from build123d import *

# Parameters (mm, degrees)
SCHIZZO1_R                   = 4
ESTRUSIONE_ESTRUSIONE1_DEPTH = 3
ESTRUSIONE_ESTRUSIONE2_DEPTH = 14
SCHIZZO3_R                   = 1.5
TAGLIO_ESTRUSIONE1_DEPTH     = 32


with BuildPart() as part:
    # Schizzo1 → Estrusione-Estrusione1 (new body)
    with BuildSketch(Plane(origin=(0, 0, 0), x_dir=(1, 0, 0), z_dir=(0, 1, 0))):
        with Locations(Location((0, 0, 0), (0, 0, 270))):
            Circle(SCHIZZO1_R)
    extrude(amount=ESTRUSIONE_ESTRUSIONE1_DEPTH)

    # Schizzo2 → Estrusione-Estrusione2 (add)
    with BuildSketch(Plane(origin=(0, 3, 0), x_dir=(1, 0, 0), z_dir=(0, 1, 0))):
        with BuildLine():
            Line((5.877166346, 8.476701011), (1.77302735, 3.585578617))
            ThreePointArc((1.77302735, 3.585578617), (1.368080573, 3.758770483), (0.94654776, 3.886392587))
            Line((0.94654776, 3.886392587), (0.94654776, 10.271299413))
            Line((0.94654776, 10.271299413), (2, 11.324751653))
            Line((2, 11.324751653), (-2, 11.324751653))
            Line((-2, 11.324751653), (-0.94654776, 10.271299413))
            Line((-0.94654776, 10.271299413), (-0.94654776, 3.886392587))
            ThreePointArc((-0.94654776, 3.886392587), (-1.368080573, 3.758770483), (-1.77302735, 3.585578617))
            Line((-1.77302735, 3.585578617), (-5.877166346, 8.476701011))
            Line((-5.877166346, 8.476701011), (-5.747321159, 9.960838293))
            Line((-5.747321159, 9.960838293), (-8.811498932, 7.389687854))
            Line((-8.811498932, 7.389687854), (-7.327361649, 7.259842667))
            Line((-7.327361649, 7.259842667), (-3.223222653, 2.368720273))
            ThreePointArc((-3.223222653, 2.368720273), (-3.464101615, 2), (-3.662983257, 1.607032563))
            Line((-3.662983257, 1.607032563), (-9.950889001, 2.715759998))
            Line((-9.950889001, 2.715759998), (-10.805406873, 3.936137993))
            Line((-10.805406873, 3.936137993), (-11.499999584, -0.003093019))
            Line((-11.499999584, -0.003093019), (-10.279621589, 0.851424853))
            Line((-10.279621589, 0.851424853), (-3.991715844, -0.257302582))
            ThreePointArc((-3.991715844, -0.257302582), (-3.939231012, -0.694592711), (-3.838988589, -1.123461888))
            Line((-3.838988589, -1.123461888), (-9.368480101, -4.315915301))
            Line((-9.368480101, -4.315915301), (-10.807522623, -3.930325019))
            Line((-10.807522623, -3.930325019), (-8.807522623, -7.394426634))
            Line((-8.807522623, -7.394426634), (-8.421932341, -5.955384112))
            Line((-8.421932341, -5.955384112), (-2.892440829, -2.762930699))
            ThreePointArc((-2.892440829, -2.762930699), (-2.571150439, -3.064177772), (-2.218688495, -3.328276035))
            Line((-2.218688495, -3.328276035), (-4.402455242, -9.328125863))
            Line((-4.402455242, -9.328125863), (-5.752678425, -9.957745274))
            Line((-5.752678425, -9.957745274), (-1.993907942, -11.325825847))
            Line((-1.993907942, -11.325825847), (-2.623527352, -9.975602664))
            Line((-2.623527352, -9.975602664), (-0.439760605, -3.975752836))
            ThreePointArc((-0.439760605, -3.975752836), (0, -4), (0.439760605, -3.975752836))
            Line((0.439760605, -3.975752836), (2.623527352, -9.975602664))
            Line((2.623527352, -9.975602664), (1.993907942, -11.325825847))
            Line((1.993907942, -11.325825847), (5.752678425, -9.957745274))
            Line((5.752678425, -9.957745274), (4.402455242, -9.328125863))
            Line((4.402455242, -9.328125863), (2.218688495, -3.328276035))
            ThreePointArc((2.218688495, -3.328276035), (2.571150439, -3.064177772), (2.892440829, -2.762930699))
            Line((2.892440829, -2.762930699), (8.421932341, -5.955384112))
            Line((8.421932341, -5.955384112), (8.807522623, -7.394426634))
            Line((8.807522623, -7.394426634), (10.807522623, -3.930325019))
            Line((10.807522623, -3.930325019), (9.368480101, -4.315915301))
            Line((9.368480101, -4.315915301), (3.838988589, -1.123461888))
            ThreePointArc((3.838988589, -1.123461888), (3.939231012, -0.694592711), (3.991715844, -0.257302582))
            Line((3.991715844, -0.257302582), (10.279621589, 0.851424853))
            Line((10.279621589, 0.851424853), (11.499999584, -0.003093019))
            Line((11.499999584, -0.003093019), (10.805406873, 3.936137993))
            Line((10.805406873, 3.936137993), (9.950889001, 2.715759998))
            Line((9.950889001, 2.715759998), (3.662983257, 1.607032563))
            ThreePointArc((3.662983257, 1.607032563), (3.464101615, 2), (3.223222653, 2.368720273))
            Line((3.223222653, 2.368720273), (7.327361649, 7.259842667))
            Line((7.327361649, 7.259842667), (8.811498932, 7.389687854))
            Line((8.811498932, 7.389687854), (5.747321159, 9.960838293))
            Line((5.747321159, 9.960838293), (5.877166346, 8.476701011))
        make_face()
    extrude(amount=ESTRUSIONE_ESTRUSIONE2_DEPTH)

    # Schizzo3 → Taglio-Estrusione1 (cut)
    with BuildSketch(Plane(origin=(0, 17, 0), x_dir=(1, 0, 0), z_dir=(0, 1, 0))):
        with Locations(Location((0, 0, 0), (0, 0, 270))):
            Circle(SCHIZZO3_R)
    extrude(amount=-TAGLIO_ESTRUSIONE1_DEPTH, mode=Mode.SUBTRACT)


solid = part.part
Input: part model. Units: mm. Frame: model coordinates. A direction names the side the tool comes from. Give positions to 0.01 mm unless a question says otherwise; leave off trailing zeros. Loops run counter-clockwise (first coordinate to the right, second up) from the corner with the lowest first, then second, coordinate; pieces in that order, holes last. Notation, with made-up numbers: M 71,68.5 L 126,68.5 A24 cw 126,105.5 Z; hole C -24,8.25 d7. An arc over 180 degrees is marked long. Use CSV: the item, a comma, the result in double quotes.
(1) Section A-A, the plane x = 0. Return loops of the section in (y, z), plus the area to 3 significant figures.
Outcome:
outline,"M 0,-4 L 3,-4 L 3,-11.32 L 17,-11.32 L 17,-1.5 L 0,-1.5 Z; M 0,1.5 L 17,1.5 L 17,4 L 0,4 Z"
area,"188 mm²"
(2) Section C-C, the plane x = -5. Return loops of the section in (y, z).
Outcome:
outline,"M 3,-7.43 L 17,-7.43 L 17,-4.49 L 3,-4.49 Z; M 3,-1.84 L 17,-1.84 L 17,0.08 L 3,0.08 Z; M 3,1.79 L 17,1.79 L 17,3.98 L 3,3.98 Z; M 3,9.61 L 17,9.61 L 17,10.23 L 3,10.23 Z"
(3) Section B-B, the plane z = -6.5. Return loops of the section in (x, y).
Outcome:
outline,"M -6.69,3 L -4.22,3 L -4.22,17 L -6.69,17 Z; M -0.95,3 L 0.95,3 L 0.95,17 L -0.95,17 Z; M 4.22,3 L 6.69,3 L 6.69,17 L 4.22,17 Z"
(4) Pull-direction query (X, two-part tool) for faces 1 (the face through (-1.481, 9.902, -10.805)), 2 (the face through (11.158, 9.902, -1.939)), 3 (the face through (-7.18, 9.902, -0.305)); classes: pulls with the +X half, pulls with the -X half, needs draft (parallel to the pull), parting line crosses it, or undercut.
Outcome:
face 1,"pulls with the -X half"
face 2,"pulls with the +X half"
face 3,"undercut"
(5) Set-up query: faces 4 (the face through (1.516, 9.902, 6.934)), 5 (the face through (8.059, 9.902, -7.324)), 6 (the face through (5, 3, -6)). Return all of +Z, -Z, +X, -X, +Y, -Y with unobstructed straight access to the full face (end or side cutting, diameter ignored); none if empty.
Outcome:
face 4,"+Y, -Y"
face 5,"+X, +Y, -Y"
face 6,"-Z, +X, -Y"
(6) Section D-D, the plane z = -0.5. Return loops of the section in (x, y), plus the area to 3 significant figures.
Outcome:
outline,"M -11.41,3 L -10.78,3 L -10.78,17 L -11.41,17 Z; M -8.29,3 L -3.97,3 L -3.97,0 L -1.41,0 L -1.41,17 L -8.29,17 Z; M 1.41,0 L 3.97,0 L 3.97,3 L 8.29,3 L 8.29,17 L 1.41,17 Z; M 10.78,3 L 11.41,3 L 11.41,17 L 10.78,17 Z"
area,"225 mm²"
(7) Pin query (flat end, axial travel): P1, Ø5, axis at x = 0, y = 2, coming from the +Z side; P2, Ø5, axis at y = 12, z = -5.5, coming from the -X side; P3, Ø2, axis at x = 8.5, z = -2.5, coming from the -Y side; P4, Ø3, axis at y = 9, z = 4, coming from the -X side. Return the tip coordinate at first contact, or that it passes through.
Outcome:
P1,"stops at z = 11.33"
P2,"stops at x = -10.97"
P3,"stops at y = 3"
P4,"stops at x = -10.81"
(8) Material intervals for L1, parallel to X at y = 12, z = -9.5; L2, parallel to Z at x = -5, y = 12; L3, parallel to Z at x = -4.75, y = 15, sorted ascending. Write a range as [from, to].
Outcome:
L1,"x = [-6.3, -5.79], [-0.95, 0.95], [5.79, 6.3]"
L2,"z = [-7.43, -4.49], [-1.84, 0.08], [1.79, 3.98], [9.61, 10.23]"
L3,"z = [-7.13, -4.19], [-1.8, 0.12], [1.65, 3.84], [9.49, 10.32]"
